from build123d import *

# Parameters (mm, degrees)
F_20_MCAT_BPL2_PCB_OUTLINE_R = 1.1
BOSS_EXTRUDE1_DEPTH          = 1.5748


with BuildPart() as part:
    # 20 MCAT BPL2 PCB Outline → Boss-Extrude1 (new body)
    with BuildSketch(Plane.XY):
        with BuildLine():
            Line((0, -53.15), (0, 0))
            Line((0, 0), (60, 0))
            ThreePointArc((60, 0), (63.535533906, -1.464466094), (65, -5))
            Line((65, -5), (65, -48.15))
            ThreePointArc((65, -48.15), (63.535533906, -51.685533906), (60, -53.15))
            Line((60, -53.15), (0, -53.15))
        make_face()
        with Locations((3, -44.15)):
            Circle(F_20_MCAT_BPL2_PCB_OUTLINE_R, mode=Mode.SUBTRACT)
        with Locations((62, -30.575)):
            Circle(F_20_MCAT_BPL2_PCB_OUTLINE_R, mode=Mode.SUBTRACT)
        with Locations((3, -9)):
            Circle(F_20_MCAT_BPL2_PCB_OUTLINE_R, mode=Mode.SUBTRACT)
        with Locations((62, -22.575)):
            Circle(F_20_MCAT_BPL2_PCB_OUTLINE_R, mode=Mode.SUBTRACT)
    extrude(amount=-BOSS_EXTRUDE1_DEPTH)


solid = part.part
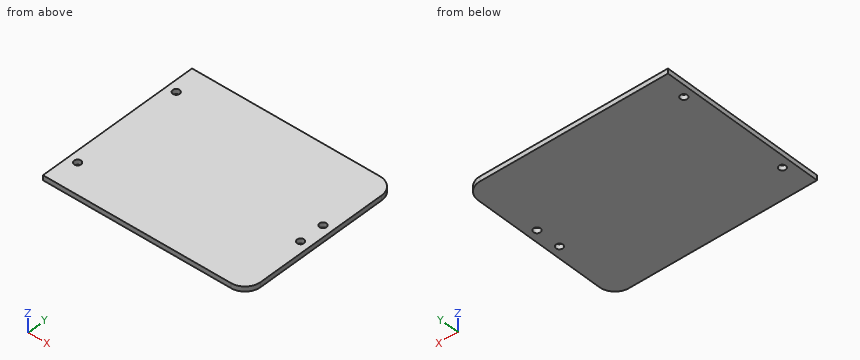
The model under review builds one solid part; all positions refer to its coordinate system, in mm. Round coordinates to 2 decimals unless told otherwise and drop trailing zeros. Write each loop counter-clockwise with the first axis right and the second up, starting at its lowest first coordinate (ties: lowest second). Pieces come first, ordered by that corner, then holes. Notation, with made-up numbers: M -7.5,23 L 7.5,23 A12 cw 7.5,38 Z; hole C -13,-38 d5. An arc over 180 degrees is marked long. Use a Markdown table: item, result. Add a question column.
Q1. To check wall thickness, follow line 1 (X direction, y = -22.5, z = -1.45); line 2 (Y direction, x = 62, z = -0.5) (3 decimals); line 3 (X direction, y = -31.5, z = -0.05). State the ranges of each line that lie inside material, in increasing order.
Q2. Insertion check: pin 1 (2 mm diameter, centred on x = 37, y = -6, fed in from +Z). The pin has a flat end and moves straight along its axis. Give the tip position at first contact, or say it passes through.
Q3. We need section C-C, the plane x = 62. State the section outline as (y, z) points (3 decimals), plus the area to 3 significant figures.
Q4. We need section A-A, the plane x = 3. State the section outline as (y, z) points.
Q5. We need section B-B, the plane y = -9. State the section outline as (x, z) points, plus the area to 3 significant figures.
Findings below:
| question | item | result |
|---|---|---|
| 1 | line 1 | x = 0 to 60.9, 63.1 to 65 |
| 1 | line 2 | y = -52.733 to -31.675, -29.475 to -23.675, -21.475 to -0.417 |
| 1 | line 3 | x = 0 to 61.4, 62.6 to 65 |
| 2 | pin 1 | stops at z = 0 |
| 3 | outline | M -52.733,-1.575 L -31.675,-1.575 L -31.675,0 L -52.733,0 Z; M -29.475,-1.575 L -23.675,-1.575 L -23.675,0 L -29.475,0 Z; M -21.475,-1.575 L -0.417,-1.575 L -0.417,0 L -21.475,0 Z |
| 3 | area | 75.5 mm² |
| 4 | outline | M -53.15,-1.57 L -45.25,-1.57 L -45.25,0 L -53.15,0 Z; M -43.05,-1.57 L -10.1,-1.57 L -10.1,0 L -43.05,0 Z; M -7.9,-1.57 L 0,-1.57 L 0,0 L -7.9,0 Z |
| 5 | outline | M 0,-1.57 L 1.9,-1.57 L 1.9,0 L 0,0 Z; M 4.1,-1.57 L 65,-1.57 L 65,0 L 4.1,0 Z |
| 5 | area | 98.9 mm² |
